Verification items for the finished model (mm, model axes). Face numbers are marked on the shaded views. A direction names the side the tool comes from. Give positions to 0.01 mm unless a question says otherwise; leave off trailing zeros. Write each loop counter-clockwise with the first axis right and the second up, starting at its lowest first coordinate (ties: lowest second). Pieces come first, ordered by that corner, then holes. Notation, with made-up numbers: (79, 40.25) - (137, 40.25) arc R16 ccw to (137, 65.25) - close; hole circle Ø10 at (84, -34.5). An arc over 180 degrees is marked (long way). Put each result on its own line as item: value.
from build123d import *

# Parameters (mm, degrees)
F3_DEPTH = 4.85


with BuildPart() as f3:
    # F2 (on Top) → F3 (new body)
    with BuildSketch(Plane.XY):
        with BuildLine():
            Line((7.9375, 24.907028094), (-3.175, 24.907028094))
            ThreePointArc((-3.175, 24.907028094), (-9.9101920908, 22.1172201848), (-12.7, 15.382028094))
            Line((-12.7, 15.382028094), (-12.7, -22.717971906))
            ThreePointArc((-12.7, -22.717971906), (-9.8802997587, -25.8730292877), (-6.4295199487, -23.4241080485))
            ThreePointArc((-6.4295199487, -23.4241080485), (-6.1376092102, -22.6929936641), (-5.6358581606, -22.0863751625))
            Line((-5.6358581606, -22.0863751625), (-2.54, -19.3483561519))
            Line((-2.54, -19.3483561519), (-4.5457479551, -17.0804715423))
            ThreePointArc((-4.5457479551, -17.0804715423), (-5.2240286378, -15.1094818757), (-4.3099453491, -13.2361648465))
            Line((-4.3099453491, -13.2361648465), (-2.54, -11.6708011372))
            Line((-2.54, -11.6708011372), (-4.4670308393, -9.4919213974))
            ThreePointArc((-4.4670308393, -9.4919213974), (-5.1749040056, -7.4349400744), (-4.2209404794, -5.4798927161))
            Line((-4.2209404794, -5.4798927161), (-2.54, -3.9932461226))
            Line((-2.54, -3.9932461226), (-5.4503163021, -0.702572669))
            ThreePointArc((-5.4503163021, -0.702572669), (-6.1175435561, 0.4027397661), (-6.35, 1.6727286595))
            Line((-6.35, 1.6727286595), (-6.35, 15.382028094))
            ThreePointArc((-6.35, 15.382028094), (-3.175, 18.557028094), (0, 15.382028094))
            Line((0, 15.382028094), (0, -22.717971906))
            ThreePointArc((0, -22.717971906), (3.175, -25.892971906), (6.35, -22.717971906))
            Line((6.35, -22.717971906), (6.35, -5.842971906))
            ThreePointArc((6.35, -5.842971906), (6.9357864376, -4.4287583436), (8.35, -3.842971906))
            Line((8.35, -3.842971906), (9.525, -3.842971906))
            ThreePointArc((9.525, -3.842971906), (13.7247767679, -1.417971906), (9.525, 1.007028094))
            Line((9.525, 1.007028094), (8.35, 1.007028094))
            ThreePointArc((8.35, 1.007028094), (6.9357864376, 1.5928145316), (6.35, 3.007028094))
            Line((6.35, 3.007028094), (6.35, 18.057028094))
            ThreePointArc((6.35, 18.057028094), (6.9357864376, 19.4712416564), (8.35, 20.057028094))
            Line((8.35, 20.057028094), (7.9375, 20.057028094))
            ThreePointArc((7.9375, 20.057028094), (13.612031919, 22.407496175), (15.9625, 28.082028094))
            Line((15.9625, 28.082028094), (15.9625, 31.257028094))
            ThreePointArc((15.9625, 31.257028094), (13.5375, 33.682028094), (11.1125, 31.257028094))
            Line((11.1125, 31.257028094), (11.1125, 28.082028094))
            ThreePointArc((11.1125, 28.082028094), (10.1825640303, 25.8369640637), (7.9375, 24.907028094))
        make_face()
    extrude(amount=F3_DEPTH)


solid = f3.part
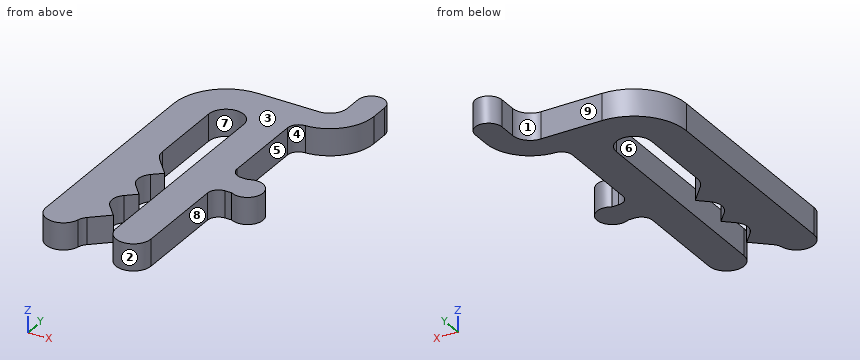
Q1. Go/stop test with flat-tipped pins: pin 1 Ø0.6 at (x, z) = (8.5, 1.5) entering from +Y; pin 2 Ø1 at (x, z) = (1, 2.5) entering from +Y; pin 3 Ø1.5 at (y, z) = (10, 3) entering from +X. Record where each tip stops, or that it passes through.
Answers follow:
pin 1: stops at y = 25.03
pin 2: stops at y = 24.91
pin 3: stops at x = 6.35
Q2. Release check for a two-part mould opening along X. For the marked faces 1, 2, 3 and 4 record: released by +X, released by -X, zero draft, split by the parting line, or undercut.
Answers follow:
face 1: released by -X
face 2: undercut
face 3: zero draft
face 4: released by +X
Q3. Section check D-D, the plane x = 1.25. Record the cut outline in (y, z).
Answers follow:
outline: (-25.24, 0) - (24.91, 0) - (24.91, 4.85) - (-25.24, 4.85) - close
Q4. Scan lines: line 1 along X through (y, z) = (-15, 0.5); line 2 along Y through (x, z) = (-3.5, 1.7); line 3 along X through (y, z) = (3, 1.4). Record each from-to range of solid material in increasing order.
Answers follow:
line 1: x = -12.7 to -5.22, 0 to 6.35
line 2: y = -20.2 to -18.26, -12.52 to -10.59, -4.84 to -2.91, 18.54 to 24.9
line 3: x = -12.7 to -6.35, 0 to 6.35
Q5. Section check B-B, the plane x = 12.75. Record the cut outline in (y, z).
Answers follow:
outline: (-3.54, 0) - (0.71, 0) - (0.71, 4.85) - (-3.54, 4.85) - close; (21.66, 0) - (33.55, 0) - (33.55, 4.85) - (21.66, 4.85) - close
Q6. Section check A-A, the plane y = 14.5. Record the cut outline in (x, z), plus the area to 3 significant figures.
Answers follow:
outline: (-12.7, 0) - (-6.35, 0) - (-6.35, 4.85) - (-12.7, 4.85) - close; (0, 0) - (6.35, 0) - (6.35, 4.85) - (0, 4.85) - close
area: 61.6 mm2
Q7. Set-up check for the marked faces 5, 6, 7, 8 and 9: record each of +Z, -Z, +X, -X, +Y, -Y from which the full face is reachable in a straight line by a thin tool's end or side.
Answers follow:
face 5: +Z, -Z, +X
face 6: +Z, -Z, -Y
face 7: +Z, -Z
face 8: +Z, -Z, +X, -Y
face 9: +Z, -Z, -X, +Y
